```python
from build123d import *

# Parameters (mm, degrees)
SKETCH1_R           = 5
BOSS_EXTRUDE1_DEPTH = 1


with BuildPart() as part:
    # Sketch1 → Boss-Extrude1 (new body)
    with BuildSketch(Plane(origin=(0, 0, 0), x_dir=(1, 0, 0), z_dir=(0, 1, 0))):
        with Locations(Location((0, 0, 0), (0, 0, 270))):
            Circle(SKETCH1_R)
        with BuildLine():
            Line((0.5, 1.936491673), (0.5, 3.5))
            Line((0.5, 3.5), (-0.5, 3.5))
            Line((-0.5, 3.5), (-0.5, 1.936491673))
            ThreePointArc((-0.5, 1.936491673), (-2, 0), (-0.5, -1.936491673))
            Line((-0.5, -1.936491673), (-0.5, -3.5))
            Line((-0.5, -3.5), (0.5, -3.5))
            Line((0.5, -3.5), (0.5, -1.936491673))
            ThreePointArc((0.5, -1.936491673), (2, 0), (0.5, 1.936491673))
        make_face(mode=Mode.SUBTRACT)
    extrude(amount=BOSS_EXTRUDE1_DEPTH)


solid = part.part
```
Design review of the part built by this model. Coordinates are the model's own, in mm. A direction names the side the tool comes from. Coordinates: 2 decimals unless noted, no trailing zeros. Write each loop counter-clockwise with the first axis right and the second up, starting at its lowest first coordinate (ties: lowest second). Pieces come first, ordered by that corner, then holes.
1) Machinability: for faces 1 (the flat face through (0, 0.5, 3.5)), 2 (the flat face through (-2.2, 0, -0.1)), which of the approach directions +Z, -Z, +X, -X, +Y, -Y give a long, thin tool a straight path to every point of the face, cutting with its end or side? Answer none if there is none.
2) Add section B-B (y = 0.35). Write out the cut boundary in (x, z).
3) Add section A-A (z = 0). Write out the cut boundary in (x, y).
4) To check wall thickness, follow L1, parallel to X at y = 0.9, z = -2.25; L2, parallel to X at y = 0.4, z = -2.75; L3, parallel to Z at x = -0.25, y = 0.55. State the ranges of each line that lie inside material, in increasing order.
5) Add section C-C (x = 0). Write out the cut boundary in (y, z).
6) Add section D-D (x = 2.75). Write out the cut boundary in (y, z).
7) Insertion check: pin 1 (0.5 mm diameter, centred on y = 0.5, z = 3, fed in from +X); pin 2 (0.5 mm diameter, centred on y = 0.5, z = 3, fed in from -X). Each pin has a flat end and moves straight along its axis. Give the tip position at first contact, or say it passes through.
8) Mouldability with a two-part tool opening along X and no side actions: class faces 3 (the flat face through (-2.2, 1, -0.1)), 4 (the cylindrical face through (-4.88, 0.49, -1.08)), 5 (the flat face through (0.5, 0.5, -2.7)) as +X half, -X half, draft (parallel to the pull), parting line (faces both ways), or undercut.
Check result:
1. face 1: +Y, -Y
1. face 2: +Z, -Z, +X, -X, -Y
2. outline: circle Ø10 at (0, 0); hole (-0.5, -3.5) - (0.5, -3.5) - (0.5, -1.94) arc R2 ccw to (0.5, 1.94) - (0.5, 3.5) - (-0.5, 3.5) - (-0.5, 1.94) arc R2 ccw to (-0.5, -1.94) - close
3. outline: (-5, 0) - (-2, 0) - (-2, 1) - (-5, 1) - close; (2, 0) - (5, 0) - (5, 1) - (2, 1) - close
4. L1: x = -4.47 to -0.5, 0.5 to 4.47
4. L2: x = -4.18 to -0.5, 0.5 to 4.18
4. L3: z = -4.99 to -3.5, 3.5 to 4.99
5. outline: (0, -5) - (1, -5) - (1, -3.5) - (0, -3.5) - close; (0, 3.5) - (1, 3.5) - (1, 5) - (0, 5) - close
6. outline: (0, -4.18) - (1, -4.18) - (1, 4.18) - (0, 4.18) - close
7. pin 1: stops at x = 4.18
7. pin 2: stops at x = -4.18
8. face 3: draft
8. face 4: parting line
8. face 5: undercut
